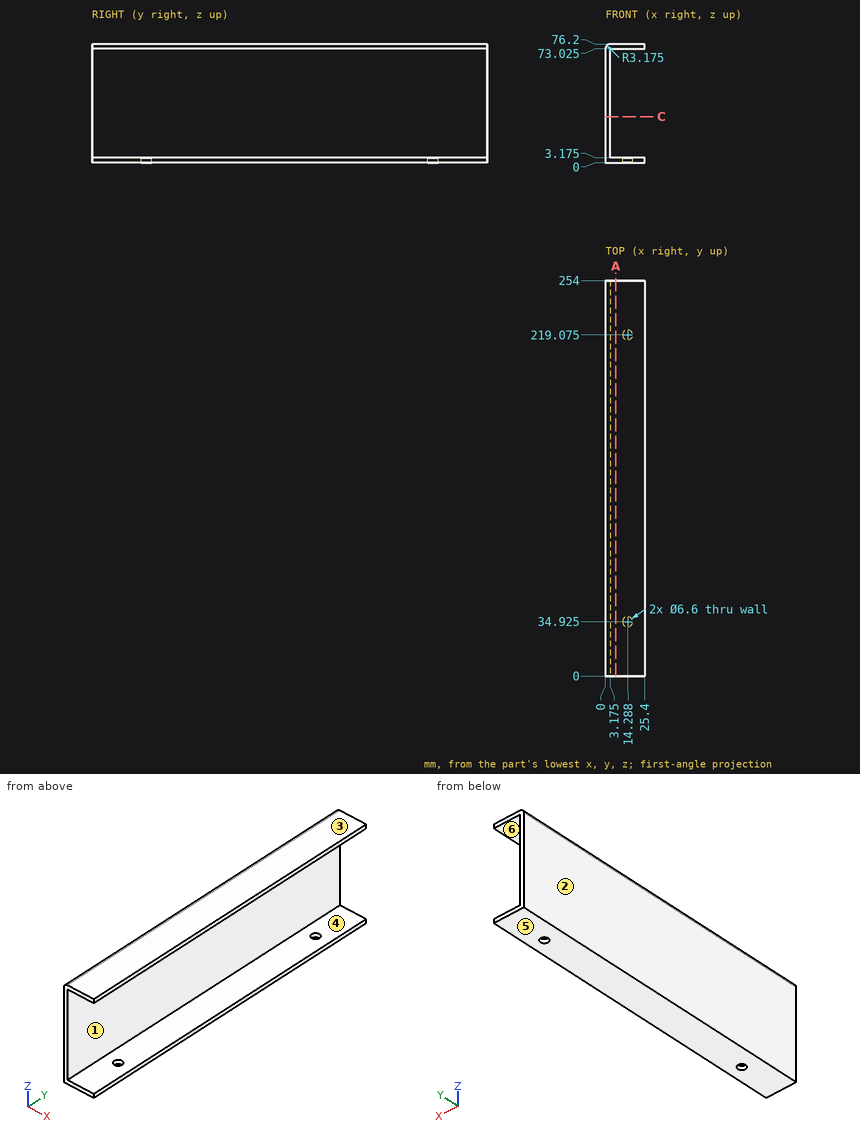
The drawing under review shows one solid part. Ordinate dimensions are in mm from its lowest x, y, z. A direction names the side the tool comes from. Give positions to 0.01 mm unless a question says otherwise; leave off trailing zeros. Loops run counter-clockwise (first coordinate to the right, second up) from the corner with the lowest first, then second, coordinate; pieces in that order, holes last. Notation, with made-up numbers: M -36,28.25 L 18,28.25 A6 cw 18,38.25 Z; hole C 79,74.5 d11. An arc over 180 degrees is marked long. One line per item, written item: value. Start each with the question number.
Q1. For L1, parallel to Z at x = 15, y = 208.5 (1 decimal); L2, parallel to X at y = 146, z = 45 (1 decimal), list the stretches that pass through material, from the lowest coordinate up.
Q2. Add section C-C (z = 29.5). Give the boundary of the cut face in (x, y) (1 decimal).
Q3. Machinability: for the marked faces 5 and 6, which of the approach directions +Z, -Z, +X, -X, +Y, -Y give a long, thin tool a straight path to every point of the face, cutting with its end or side? Answer none if there is none.
Q4. Add section A-A (x = 6.75). Give the boundary of the cut face in (y, z) (1 decimal).
Q5. Clearance check with flat-ended pins moving along their axes: pin 1 Ø4 at (x, y) = (14.29, 219.08) entering from -Z (1 decimal); pin 2 Ø6 at (y, z) = (225, 62) entering from +X (1 decimal). State where each tip first meets the part, or that it passes through.
Q6. Draft analysis for pull direction Z (two halves, no side actions). For the marked faces 1, 2, 3 and 4, state which applies: released by +Z, released by -Z, zero draft, split by the parting line, or undercut.
Reply:
1. L1: 0 to 3.2, 73 to 76.2
1. L2: 0 to 3.2
2. outline: M 0,0 L 3.2,0 L 3.2,254 L 0,254 Z
3. face 5: -Z, +X, -X, +Y, -Y
3. face 6: +X, +Y, -Y
4. outline: M 0,0 L 254,0 L 254,3.2 L 0,3.2 Z; M 0,73 L 254,73 L 254,76.2 L 0,76.2 Z
5. pin 1: z = 73
5. pin 2: x = 3.2
6. face 1: undercut
6. face 2: zero draft
6. face 3: released by +Z
6. face 4: undercut
